from build123d import *

# Parameters (mm, degrees)
BOSS_EXTRUDE1_DEPTH = 50
SKETCH2_R           = 10
CUT_EXTRUDE1_DEPTH  = 77
SCALE1_SCALE        = 0.75
SKETCH4_W           = 30
SKETCH4_H           = 50
CUT_EXTRUDE2_DEPTH  = 18.75


with BuildPart() as part:
    # Sketch1 → Boss-Extrude1 (new body)
    with BuildSketch(Plane(origin=(0, 0, 0), x_dir=(1, 0, 0), z_dir=(0, 1, 0))):
        Polygon((50, -77.599909443), (120, -147.599909443), (50, -147.599909443), (-20, -147.599909443), (-20, 102.400090557), (20, 102.400090557), (20, -77.599909443), align=None)
    extrude(amount=BOSS_EXTRUDE1_DEPTH)

    # Sketch2 → Cut-Extrude1 (cut)
    with BuildSketch(Plane(origin=(0, 50, 0), x_dir=(1, 0, 0), z_dir=(0, 1, 0))):
        with Locations(Location((0, 82.400090557, 0), (0, 0, 270))):
            Circle(SKETCH2_R)
    extrude(amount=-CUT_EXTRUDE1_DEPTH, mode=Mode.SUBTRACT)


with BuildPart() as part_1:
    # Scale1: scaled about (17.783752388, 25, 55.690336976)
    add(part.part.scale(SCALE1_SCALE).moved(Location((4.445938097, 6.25, 13.922584244))))

    # Sketch4 → Cut-Extrude2 (cut)
    with BuildSketch(Plane(origin=(0, 43.75, 0), x_dir=(1, 0, 0), z_dir=(0, 1, 0))):
        with Locations((4.445938097, 37.877483673)):
            Rectangle(SKETCH4_W, SKETCH4_H)
    extrude(amount=-CUT_EXTRUDE2_DEPTH, mode=Mode.SUBTRACT)


solid = part_1.part
For this review, take the finished solid that the model builds, in its own axes (mm). A direction names the side the tool comes from. Round coordinates to 2 decimals unless told otherwise and drop trailing zeros. Write each loop counter-clockwise with the first axis right and the second up, starting at its lowest first coordinate (ties: lowest second). Pieces come first, ordered by that corner, then holes. Notation, with made-up numbers: (5, 60) -> (34, 60) arc R20 cw to (34, 68) -> close; hole circle Ø1 at (68.25, 58). An arc over 180 degrees is marked (long way). Put each result on its own line as item: value.
Q1. The part is to be moulded in two halves that separate along X. For faces 1 (the cylindrical face through (6.699, 15.756, -40.724)), 2 (the flat face through (4, 15, -62.877)), 3 (the flat face through (-10.554, 25, 32)), say which applies: released by +X, released by -X, zero draft, split by the parting line, or undercut.
Determined:
face 1: undercut
face 2: zero draft
face 3: released by -X
Q2. To check wall thickness, follow L1, parallel to X at y = 11, z = -29.5; L2, parallel to Z at x = 27.5, y = 17; L3, parallel to X at y = 13, z = -52. State the ranges of each line that lie inside material, in increasing order. Write a range as [from, to].
Determined:
L1: x = [-10.55, 19.45]
L2: z = [72.12, 124.62]
L3: x = [-10.55, -1.82], [10.71, 19.45]
Q3. Consider section B-B on y = 18. State the section outline as (x, z) points, and give its area (3 significant figures).
Determined:
outline: (-10.55, -62.88) -> (19.45, -62.88) -> (19.45, 72.12) -> (41.95, 72.12) -> (94.45, 124.62) -> (-10.55, 124.62) -> close; hole circle Ø15 at (4.45, -47.88)
area: 8,010 mm^2
Q4. Clearance check with flat-ended pins moving along their axes: pin 1 Ø12 at (x, z) = (4.45, -47.88) entering from +Y; pin 2 Ø2 at (y, z) = (29.5, 94) entering from +X; pin 3 Ø19 at (y, z) = (17, -21) entering from +X; pin 4 Ø7 at (x, y) = (32, 25) entering from -Z. State where each tip first meets the part, or that it passes through.
Determined:
pin 1: passes through
pin 2: stops at x = 64.82
pin 3: stops at x = 19.45
pin 4: stops at z = 72.12
Q5. Consider section A-A on x = 9. State the section outline as (y, z) points.
Determined:
outline: (6.25, -62.88) -> (25, -62.88) -> (25, -53.84) -> (6.25, -53.84) -> close; (6.25, -41.92) -> (25, -41.92) -> (25, -12.88) -> (43.75, -12.88) -> (43.75, 124.62) -> (6.25, 124.62) -> close
Q6. Consider section C-C on x = 24. State the section outline as (y, z) points, and give its area (3 significant figures).
Determined:
outline: (6.25, 72.12) -> (43.75, 72.12) -> (43.75, 124.62) -> (6.25, 124.62) -> close
area: 1,970 mm^2
Q7. Machinability: for faces 4 (the flat face through (4, 25, -38)), 5 (the flat face through (31, 25, 72.123)), 6 (the flat face through (41, 25, 124.623)), which of the approach directions +Z, -Z, +X, -X, +Y, -Y give a long, thin tool a straight path to every point of the face, cutting with its end or side? Answer none if there is none.
Determined:
face 4: -Z, +X, -X, +Y
face 5: -Z, +X, +Y, -Y
face 6: +Z, +X, -X, +Y, -Y
Q8. Consider section D-D on y = 32. State the section outline as (x, z) points, and give its area (3 significant figures).
Determined:
outline: (-10.55, -12.88) -> (19.45, -12.88) -> (19.45, 72.12) -> (41.95, 72.12) -> (94.45, 124.62) -> (-10.55, 124.62) -> close
area: 6,680 mm^2
